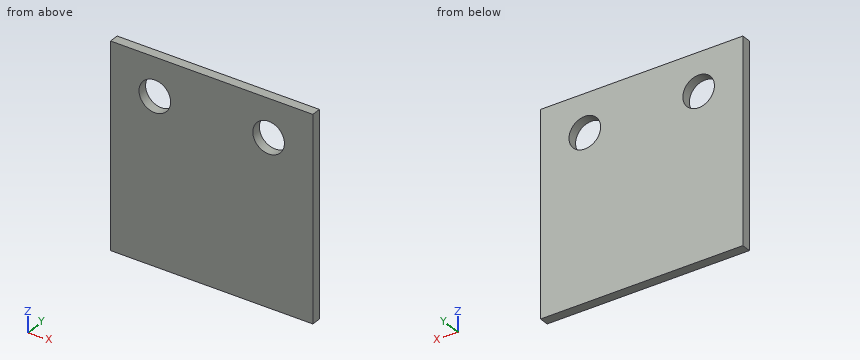
```python
from build123d import *

# Parameters (mm, degrees)
SKETCH_1_W          = 32
SKETCH_1_H          = 32
EXTRUDE_1_DEPTH     = 1.5
SKETCH_2_R          = 2.5
CUT_EXTRUDE_1_DEPTH = 23.677080941


with BuildPart() as part:
    # 草图1 → 凸台-拉伸1 (new body)
    with BuildSketch(Plane(origin=(0, 0, 0), x_dir=(1, 0, 0), z_dir=(0, 1, 0))):
        Rectangle(SKETCH_1_W, SKETCH_1_H)
    extrude(amount=EXTRUDE_1_DEPTH)

    # 草图2 → 切除-拉伸1 (cut, through all)
    with BuildSketch(Plane(origin=(0, 1.5, 0), x_dir=(1, 0, 0), z_dir=(0, 1, 0))):
        with Locations(Location((9, -10, 0), (0, 0, 270))):
            Circle(SKETCH_2_R)
    cut_extrude_1 = extrude(amount=-CUT_EXTRUDE_1_DEPTH, mode=Mode.SUBTRACT)

    # 镜向1: 切除-拉伸1 across plane
    add(cut_extrude_1.mirror(Plane(origin=(0, 0, 0), x_dir=(0, 0, 1), z_dir=(1, 0, 0))), mode=Mode.SUBTRACT)


solid = part.part
```
The listing builds one solid part. Answer for the finished solid, in the listing's coordinates (mm). Round coordinates to 2 decimals unless told otherwise and drop trailing zeros. Order: outer loops, then holes, each group sorted by start corner. A loop starts at its lowest first (then second) coordinate and runs counter-clockwise, first axis right, second up. Notation, with made-up numbers: (22, 32.5) -> (36, 32.5) arc R12 cw to (36, 40.5) -> close; hole circle Ø1 at (26, -29). An arc over 180 degrees is marked (long way). Answer as CSV lines item,"result".
Q1. Given pin 1 (4 mm diameter, centred on x = 12.5, z = -3, fed in from -Y); pin 2 (4.5 mm diameter, centred on x = 9, z = 10, fed in from -Y), each flat-ended and moving along its own axis, determine where each tip first touches the part or whether it passes through.
Computed values:
pin 1,"stops at y = 0"
pin 2,"passes through"
Q2. A cutting plane is placed at A-A on z = 10. Determine the outline of the cut face in (x, y).
Computed values:
outline,"(-16, 0) -> (-11.5, 0) -> (-11.5, 1.5) -> (-16, 1.5) -> close; (-6.5, 0) -> (6.5, 0) -> (6.5, 1.5) -> (-6.5, 1.5) -> close; (11.5, 0) -> (16, 0) -> (16, 1.5) -> (11.5, 1.5) -> close"
Q3. A cutting plane is placed at C-C on y = 0.9. Determine the outline of the cut face in (x, z), plus the area to 3 significant figures.
Computed values:
outline,"(-16, -16) -> (16, -16) -> (16, 16) -> (-16, 16) -> close; hole circle Ø5 at (-9, 10); hole circle Ø5 at (9, 10)"
area,"985 mm^2"
Q4. A cutting plane is placed at B-B on x = -9. Determine the outline of the cut face in (y, z), plus the area to 3 significant figures.
Computed values:
outline,"(0, -16) -> (1.5, -16) -> (1.5, 7.5) -> (0, 7.5) -> close; (0, 12.5) -> (1.5, 12.5) -> (1.5, 16) -> (0, 16) -> close"
area,"40.5 mm^2"
Q5. A cutting plane is placed at D-D on x = 7.5. Determine the outline of the cut face in (y, z), plus the area to 3 significant figures.
Computed values:
outline,"(0, -16) -> (1.5, -16) -> (1.5, 8) -> (0, 8) -> close; (0, 12) -> (1.5, 12) -> (1.5, 16) -> (0, 16) -> close"
area,"42.0 mm^2"
Q6. Consider line 1 (X direction, y = 0.85, z = 10); line 2 (Z direction, x = -9, y = 1); line 3 (Z direction, x = 7.5, y = 0.45). Determine where each line is inside the solid, lowest interval first. Write a range as from..to.
Computed values:
line 1,"x = -16..-11.5, -6.5..6.5, 11.5..16"
line 2,"z = -16..7.5, 12.5..16"
line 3,"z = -16..8, 12..16"
